```python
from build123d import *

# Parameters (mm, degrees)
SKETCH1_W           = 481.0125
SKETCH1_H           = 379.4125
BOSS_EXTRUDE1_DEPTH = 25.4
FILLET1_R           = 12.7
SKETCH2_W           = 22.225
SKETCH2_H           = 22.225
CUT_EXTRUDE2_DEPTH  = 25.4
SKETCH3_R           = 5.55625
CUT_EXTRUDE3_DEPTH  = 25.4


with BuildPart() as part:
    # Sketch1 → Boss-Extrude1 (new body)
    with BuildSketch(Plane(origin=(0, 0, 0), x_dir=(1, 0, 0), z_dir=(0, 1, 0))):
        with Locations((240.50625, 189.70625)):
            Rectangle(SKETCH1_W, SKETCH1_H)
    extrude(amount=BOSS_EXTRUDE1_DEPTH)

    # Fillet1
    fillet1_edges = [part.edges().sort_by_distance(p)[0] for p in [
        (0, 12.7, -379.4125),
        (481.0125, 12.7, -379.4125),
        (481.0125, 12.7, 0),
        (0, 12.7, 0),
    ]]
    fillet(fillet1_edges, radius=FILLET1_R)

    # Sketch2 → Cut-Extrude2 (cut)
    with BuildSketch(Plane(origin=(0, 25.4, 0), x_dir=(1, 0, 0), z_dir=(0, 1, 0))):
        with Locations((43.65625, 117.739583291)):
            Rectangle(SKETCH2_W, SKETCH2_H)
        with Locations((43.65625, 261.672916709)):
            Rectangle(SKETCH2_W, SKETCH2_H)
        with Locations((174.889583418, 45.772916582)):
            Rectangle(SKETCH2_W, SKETCH2_H)
        with Locations((306.122916582, 117.739583291)):
            Rectangle(SKETCH2_W, SKETCH2_H)
        with Locations((437.35625, 45.772916582)):
            Rectangle(SKETCH2_W, SKETCH2_H)
        with Locations((437.35625, 189.70625)):
            Rectangle(SKETCH2_W, SKETCH2_H)
        with Locations((437.35625, 333.639583418)):
            Rectangle(SKETCH2_W, SKETCH2_H)
        with Locations((174.889583418, 189.70625)):
            Rectangle(SKETCH2_W, SKETCH2_H)
        with Locations((174.889583418, 333.639583418)):
            Rectangle(SKETCH2_W, SKETCH2_H)
        with Locations((306.122916582, 261.672916709)):
            Rectangle(SKETCH2_W, SKETCH2_H)
    extrude(amount=-CUT_EXTRUDE2_DEPTH, mode=Mode.SUBTRACT)

    # Sketch3 → Cut-Extrude3 (cut)
    with BuildSketch(Plane(origin=(0, 25.4, 0), x_dir=(1, 0, 0), z_dir=(0, 1, 0))):
        with Locations(Location((25.4, 328.6125, 0), (0, 0, 270))):
            Circle(SKETCH3_R)
        with Locations(Location((50.8, 354.0125, 0), (0, 0, 270))):
            Circle(SKETCH3_R)
    extrude(amount=-CUT_EXTRUDE3_DEPTH, mode=Mode.SUBTRACT)


solid = part.part
```
Input: part model. Units: mm. Frame: model coordinates. A direction names the side the tool comes from. Coordinates: 2 decimals unless noted, no trailing zeros. Order: outer loops, then holes, each group sorted by start corner. A loop starts at its lowest first (then second) coordinate and runs counter-clockwise, first axis right, second up. Notation, with made-up numbers: (3, 46) - (19, 46) arc R34 cw to (19, 78) - close; hole circle Ø5 at (-30, 10). An arc over 180 degrees is marked (long way). Put each result on its own line as item: value.
1. Cut plane B-B on x = 25.4. Return the cut outline in (y, z).
Report:
outline: (0, -379.41) - (25.4, -379.41) - (25.4, -334.17) - (0, -334.17) - close; (0, -323.06) - (25.4, -323.06) - (25.4, 0) - (0, 0) - close
2. Reachability of faces 5 (the face through (186.002, 13, -190)), 6 (the face through (477.19, 12.88, -3.62)) from +Z, -Z, +X, -X, +Y, -Y: full face, straight path, thin tool, end or side. Return the list, or none.
Report:
face 5: +Y, -Y
face 6: +Z, +X, +Y, -Y
3. Line query: line 1 along X through (y, z) = (23.5, -122); line 2 along X through (y, z) = (15, -338.5); line 3 along Z through (x, y) = (52, 24.25). Output: solid intervals per line, ascending.
Report:
line 1: x = 0 to 32.54, 54.77 to 295.01, 317.24 to 481.01
line 2: x = 0 to 163.78, 186 to 426.24, 448.47 to 481.01
line 3: z = -379.41 to -359.44, -348.59 to -272.79, -250.56 to -128.85, -106.63 to 0
4. Cut plane A-A on z = -258. Return the cut outline in (x, y), then the cut area to 3 significant figures.
Report:
outline: (0, 0) - (32.54, 0) - (32.54, 25.4) - (0, 25.4) - close; (54.77, 0) - (295.01, 0) - (295.01, 25.4) - (54.77, 25.4) - close; (317.24, 0) - (481.01, 0) - (481.01, 25.4) - (317.24, 25.4) - close
area: 11,100 mm2
5. Cut plane C-C on y = 14. State how many separate pieces and enclosed holes the cut face has, then the cut area to 3 significant figures.
Report:
separate pieces: 1
enclosed holes: 12
area: 177,000 mm2
6. Draft query along X for faces 1 (the face through (237, 0, -192)), 2 (the face through (3.62, 12.88, -3.82)), 3 (the face through (306, 13, -272.785)), 4 (the face through (306, 13, -250.56)). Return one class per face: pulls with the +X half, pulls with the -X half, needs draft (parallel to the pull), parting line crosses it, or undercut.
Report:
face 1: needs draft
face 2: pulls with the -X half
face 3: undercut
face 4: undercut
